Here's how the part is built. I have some questions about the finished solid (model axes, mm). A direction names the side the tool comes from. Round coordinates to 2 decimals unless told otherwise and drop trailing zeros. Order: outer loops, then holes, each group sorted by start corner. A loop starts at its lowest first (then second) coordinate and runs counter-clockwise, first axis right, second up. Notation, with made-up numbers: (49, -33.5) -> (98, -33.5) arc R19 cw to (98, -0.5) -> close; hole circle Ø7 at (-35, 21.25). An arc over 180 degrees is marked (long way). Answer in a Markdown table with one row per item.
Autodesk Inventor part; units mm, degrees
ref_plane "YZ Plane" through (0, 0, 0) normal (1, 0, 0) x (0, 1, 0)
ref_plane "XZ Plane" through (0, 0, 0) normal (0, 1, 0) x (-1, 0, 0)
ref_plane "XY Plane" through (0, 0, 0) normal (0, 0, 1) x (1, 0, 0)
sketch "Sketch1" plane through (0, 0, 0) normal (0, 1, 0) x (-1, 0, 0)
  circle A0 centre (0, 0) radius 8
  circle A1 centre (0, 0) radius 13
  circle A2 centre (0, 0) radius 20
  circle A3 centre (0, 0) radius 25
  circle A4 centre (0, 0) radius 32
  dimension "d0" = 16
  dimension "d1" = 5
  dimension "d2" = 7
  dimension "d3" = 5
  dimension "d4" = 7
extrude "Extrusion1" add sketch "Sketch1" along normal blind 1.5 contours A0 | A1 | A2 | A3 | A4
extrude "Extrusion2" add sketch "Sketch1" along normal blind 3
properties part number "Marker1"
1. For pin 1 Ø1.5 at (y, z) = (1.5, -2) entering from +X, with a flat end and sliding along its axis, tell me the tip position at first contact or that it passes through.
Numbers:
| item | result |
|---|---|
| pin 1 | stops at x = 31.98 |
2. Suppose I cut it at A-A on y = 2.5. Write out the boundary of the cut face in (x, z).
Numbers:
| item | result |
|---|---|
| outline | circle Ø64 at (0, 0); circle Ø40 at (0, 0); circle Ø16 at (0, 0); hole circle Ø50 at (0, 0); hole circle Ø26 at (0, 0) |
3. Please list where these lines run through material, in increasing order: line 1 along Z through (x, y) = (0, 2.4); line 2 along X through (y, z) = (1.7, -14.5); line 3 along X through (y, z) = (1.55, 16.5).
Numbers:
| item | result |
|---|---|
| line 1 | z = -32 to -25, -20 to -13, -8 to 8, 13 to 20, 25 to 32 |
| line 2 | x = -28.53 to -20.37, -13.77 to 13.77, 20.37 to 28.53 |
| line 3 | x = -27.42 to -18.78, -11.3 to 11.3, 18.78 to 27.42 |
4. Suppose I cut it at D-D on z = 0. Write out the boundary of the cut face in (x, y), then the cut area to 3 significant figures.
Numbers:
| item | result |
|---|---|
| outline | (-32, 0) -> (32, 0) -> (32, 3) -> (25, 3) -> (25, 1.5) -> (20, 1.5) -> (20, 3) -> (13, 3) -> (13, 1.5) -> (8, 1.5) -> (8, 3) -> (-8, 3) -> (-8, 1.5) -> (-13, 1.5) -> (-13, 3) -> (-20, 3) -> (-20, 1.5) -> (-25, 1.5) -> (-25, 3) -> (-32, 3) -> close |
| area | 162 mm2 |
5. Suppose I cut it at B-B on x = 0. Write out the boundary of the cut face in (y, z).
Numbers:
| item | result |
|---|---|
| outline | (0, -32) -> (3, -32) -> (3, -25) -> (1.5, -25) -> (1.5, -20) -> (3, -20) -> (3, -13) -> (1.5, -13) -> (1.5, -8) -> (3, -8) -> (3, 8) -> (1.5, 8) -> (1.5, 13) -> (3, 13) -> (3, 20) -> (1.5, 20) -> (1.5, 25) -> (3, 25) -> (3, 32) -> (0, 32) -> close |
6. For faces 4 (the face through (0, 0, 0)), 5 (the face through (4.336, 2.24, 19.524)), which set-ups out of +Z, -Z, +X, -X, +Y, -Y let a thin tool reach every point of the face, with its end or its side?
Numbers:
| item | result |
|---|---|
| face 4 | +Z, -Z, +X, -X, -Y |
| face 5 | +Y |
7. Suppose I cut it at C-C on z = -24. Write out the boundary of the cut face in (x, y).
Numbers:
| item | result |
|---|---|
| outline | (-21.17, 0) -> (21.17, 0) -> (21.17, 3) -> (7, 3) -> (7, 1.5) -> (-7, 1.5) -> (-7, 3) -> (-21.17, 3) -> close |
8. We'd pull the mould along X, two halves only. Please class faces 1 (the face through (-23.846, 2.24, -7.509)), 2 (the face through (19.1, 3, -16.4)), 3 (the face through (6.94, 1.48, 31.24)): released by +X, released by -X, zero draft, split by the parting line, or undercut.
Numbers:
| item | result |
|---|---|
| face 1 | undercut |
| face 2 | zero draft |
| face 3 | split by the parting line |
